```python
from build123d import *

# Parameters (mm, degrees)
F1_DEPTH    = 19.812
F2_T1_DEPTH = 189.0971878823
F3_T1_DEPTH = 189.0971878823
F3_T3_DEPTH = 105.0231878823


# Not quite as in the source:
# - a fillet or chamfer that OpenCascade refuses, or shapes differently, is made with other operations: its cross-section is extruded or revolved along the edge and cut away or added


with BuildPart() as f1:
    # F0 (on Front) → F1 (new body)
    with BuildSketch(Plane.XZ):
        Polygon((35.306, 9.8661940299), (33.528, 10.795), (-64.516, 10.795), (-64.516, -10.795), (18.288, -10.795), (25.5529864014, -1.905), (35.306, -10.795), align=None)
        Polygon((50.546, -10.795), (50.546, 1.905), (35.306, 9.8661940299), (35.306, -10.795), align=None)
        Polygon((64.516, -10.795), (64.516, 10.795), (50.546, 10.795), (50.546, 1.905), (50.546, -10.795), align=None)
    extrude(amount=F1_DEPTH)

    # F2: chamfer of 10.16 x 17.5976362049 on 1 edges, made by hand

    # F2_s2 → F2_t1 (cut)
    with BuildSketch(Plane.YZ.offset(-110.0425939411)):
        Polygon((-9.652, 10.795), (-19.812, -6.8026362049), (-19.812, 10.795), align=None)
    extrude(amount=F2_T1_DEPTH, mode=Mode.SUBTRACT)

    # F3: chamfer of 10.16 x 17.5976362049 on 2 edges, made by hand

    # F3_s2 → F3_t1 (cut)
    with BuildSketch(Plane.YZ.offset(-110.0425939411)):
        Polygon((0, -6.8026362049), (-10.16, 10.795), (0, 10.795), align=None)
    extrude(amount=F3_T1_DEPTH, mode=Mode.SUBTRACT)

    # F3_s4 → F3_t3 (cut)
    with BuildSketch(Plane.YZ.offset(5.0194060589)):
        Polygon((0, -6.8026362049), (-10.16, 10.795), (0, 10.795), align=None)
    extrude(amount=F3_T3_DEPTH, mode=Mode.SUBTRACT)


solid = f1.part
```
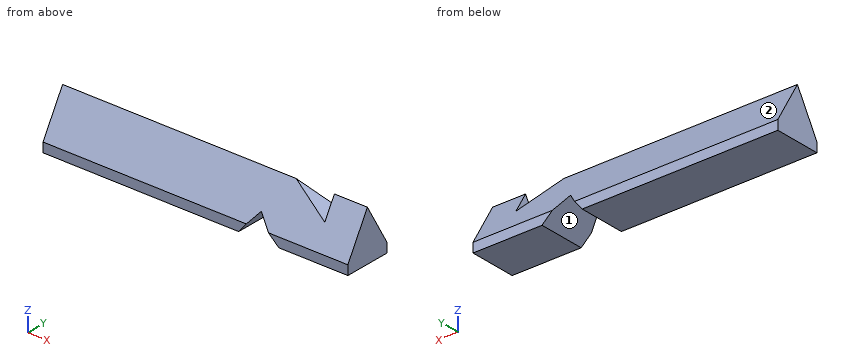
Part model, mm, in its own coordinate system. Face numbers are marked on the shaded views. A direction names the side the tool comes from. Round coordinates to 2 decimals unless told otherwise and drop trailing zeros. Loops run counter-clockwise (first coordinate to the right, second up) from the corner with the lowest first, then second, coordinate; pieces in that order, holes last.
1. 3-axis set-ups, long thin cutter, end or side, ignore diameter. For the marked faces 1 and 2: which of +Z, -Z, +X, -X, +Y, -Y reach the whole face in a straight line?
Solutions:
face 1: -Z, +Y, -Y
face 2: +Z, +X, -X, +Y
2. Slice it at A-A (z = -9.25). Give the cut face in (x, y).
Solutions:
outline: (-64.52, -19.81) - (19.55, -19.81) - (19.55, 0) - (-64.52, 0) - close; (33.61, -19.81) - (64.52, -19.81) - (64.52, 0) - (33.61, 0) - close
3. Slice it at D-D (y = -6.5). Give the cut face in (x, z) (3 decimals).
Solutions:
outline: (-64.516, -10.795) - (18.288, -10.795) - (25.553, -1.905) - (35.306, -10.795) - (64.516, -10.795) - (64.516, 4.456) - (50.546, 4.456) - (50.546, 1.905) - (45.663, 4.456) - (-64.516, 4.456) - close
4. Drill centre lines: line 1 along X through (y, z) = (-10.5, -4.75); line 2 along X through (y, z) = (-18.75, -7.5); line 3 along Y through (x, z) = (11.5, -1.75). Where is each one in solid material? Low to high.
Solutions:
line 1: x = -64.52 to 23.23, 28.67 to 64.52
line 2: x = -64.52 to 20.98, 31.69 to 64.52
line 3: y = -16.89 to -2.92
5. Slice it at C-C (x = -43). Give the cut face in (y, z) (3 decimals).
Solutions:
outline: (-19.812, -10.795) - (0, -10.795) - (0, -6.803) - (-9.906, 10.355) - (-19.812, -6.803) - close
6. Flat gauge pins, fed straight in: pin 1 (1.5 mm diameter, centred on x = -14, z = 7.5, fed in from +Y); pin 2 (4 mm diameter, centred on x = -49.5, y = -3.5, fed in from +Z); pin 3 (3 mm diameter, centred on x = -15, z = 0, fed in from +Y). Where does each tip first touch, or does it go through?
Solutions:
pin 1: stops at y = -7.82
pin 2: stops at z = 2.72
pin 3: stops at y = -3.06
7. Slice it at B-B (y = -18.5). Give the cut face in (x, z) (3 decimals).
Solutions:
outline: (-64.516, -10.795) - (18.288, -10.795) - (23.408, -4.53) - (-64.516, -4.53) - close; (28.433, -4.53) - (35.306, -10.795) - (64.516, -10.795) - (64.516, -4.53) - close
